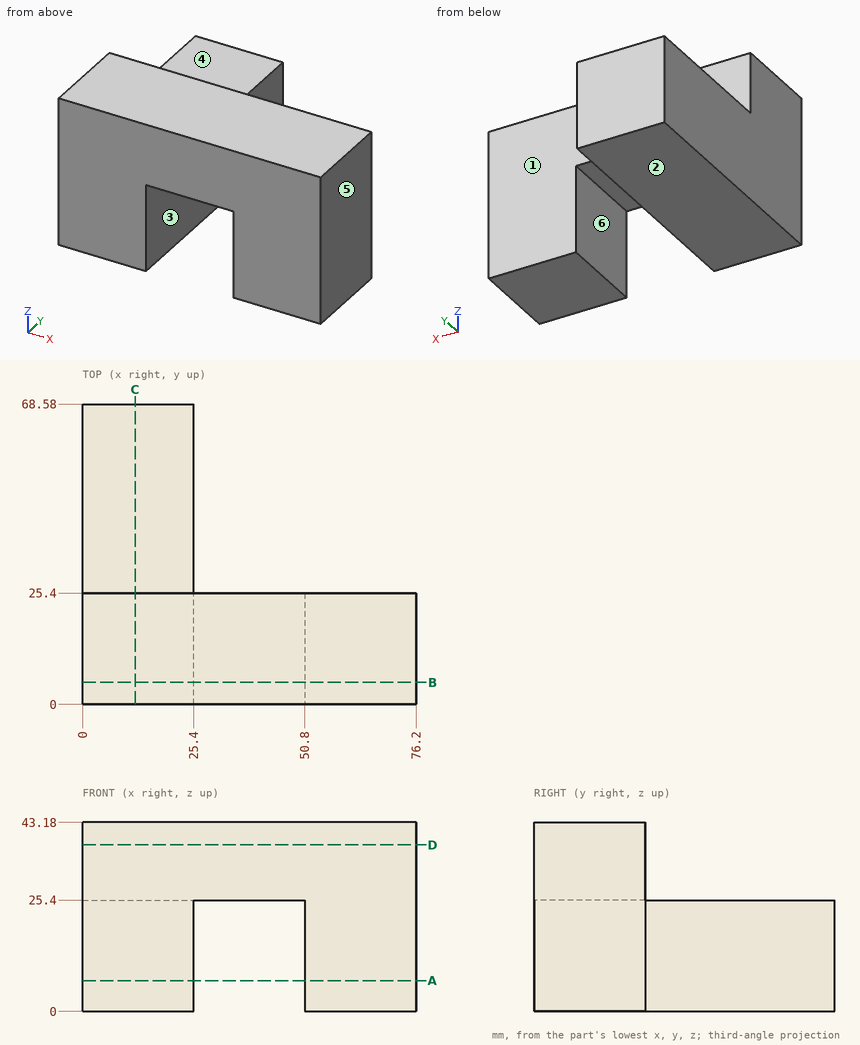
Input: dimensioned drawing with shaded views. Units: mm. Origin: part minimum x, y, z. A direction names the side the tool comes from. Coordinates: 2 decimals unless noted, no trailing zeros. Loops run counter-clockwise (first coordinate to the right, second up) from the corner with the lowest first, then second, coordinate; pieces in that order, holes last. Notation, with made-up numbers: M -31.75,77 L -3.75,77 A22 ccw -3.75,100 Z; hole C 15.5,66 d4. An arc over 180 degrees is marked long. Put each result on its own line as item: value.
(1) Access query for the marked faces 1, 2 and 3. Directions: +Z, -Z, +X, -X, +Y, -Y. A direction counts if a zero-diameter tool reaches every point of the face in a straight line with its end or side. Return the directions, or none.
Answer sheet:
face 1: +Z, +X, +Y
face 2: -Z, +X, -X, +Y, -Y
face 3: -Z, +Y, -Y
(2) Cut plane B-B on y = 5. Return the cut outline in (x, z), then the cut area to 3 significant figures.
Answer sheet:
outline: M 0,0 L 25.4,0 L 25.4,25.4 L 50.8,25.4 L 50.8,0 L 76.2,0 L 76.2,43.18 L 0,43.18 Z
area: 2,650 mm^2
(3) Material intervals for probe 1 along X at (y, z) = (16.5, 9); probe 2 along Y at (x, z) = (53.5, 37), sorted ascending.
Answer sheet:
probe 1: x = 0 to 25.4, 50.8 to 76.2
probe 2: y = 0 to 25.4
(4) Cut plane C-C on x = 12. Return the cut outline in (y, z).
Answer sheet:
outline: M 0,0 L 68.58,0 L 68.58,25.4 L 25.4,25.4 L 25.4,43.18 L 0,43.18 Z
(5) Cut plane D-D on z = 38. Return the cut outline in (x, y), then the cut area to 3 significant figures.
Answer sheet:
outline: M 0,0 L 76.2,0 L 76.2,25.4 L 0,25.4 Z
area: 1,940 mm^2
(6) First-contact query: pin 1 (20.5 mm diameter, centred on x = 36, y = 17, fed in from -Z); pin 2 (10 mm diameter, centred on x = 59, y = 34.5, fed in from -Z); pin 3 (1 mm diameter, centred on y = 26.5, z = 4.5, fed in from +X); pin 4 (6 mm diameter, centred on x = 56, z = 17, fed in from +Y). Flat tips, straight axial feed; report the tip coordinate or a pass-through.
Answer sheet:
pin 1: stops at z = 25.4
pin 2: passes through
pin 3: stops at x = 25.4
pin 4: stops at y = 25.4
(7) Draft query along X for the marked faces 4, 5 and 6. Return one class per face: pulls with the +X half, pulls with the -X half, needs draft (parallel to the pull), parting line crosses it, or undercut.
Answer sheet:
face 4: needs draft
face 5: pulls with the +X half
face 6: undercut
(8) Cut plane A-A on z = 7. Return the cut outline in (x, y).
Answer sheet:
outline: M 0,0 L 25.4,0 L 25.4,68.58 L 0,68.58 Z; M 50.8,0 L 76.2,0 L 76.2,25.4 L 50.8,25.4 Z
